Verification items for the finished model (mm, model axes). A direction names the side the tool comes from. Coordinates: 2 decimals unless noted, no trailing zeros. Order: outer loops, then holes, each group sorted by start corner. A loop starts at its lowest first (then second) coordinate and runs counter-clockwise, first axis right, second up.
Q1. Thickness scan on line 1 (X direction, y = 51, z = 1.8); line 2 (Y direction, x = 12, z = 0.2); line 3 (Y direction, x = 24, z = 1.05). Record the ranges inside material, lowest first.
Q2. Draft check along X on faces 1 (the cylindrical face through (78.084, 57.374, 0.986)), 2 (the cylindrical face through (-73.42, -0.79, 0.99)), 3 (the flat face through (1, 9, 2)). Enter one of: pulls with the +X half, pulls with the -X half, needs draft (parallel to the pull), parting line crosses it, or undercut.
Q3. Cross-section at B-B, the plane y = 51. Record the boundary of the cut face in (x, z), and give its area (3 significant figures).
Q4. Depth check by flat-ended pin: P1, Ø3.5, axis at x = 12.15, y = 85.47, coming from the +Z side; P2, Ø1, axis at y = -68, z = 1.5, coming from the +X side; P3, Ø1, axis at y = 42.5, z = 1, coming from the +X side; P4, Ø3.5, axis at x = -58.16, y = -76.19, coming from the -Z side. Enter the tip coordinate at first touch or a pass-through.
Q5. Cross-section at C-C, the plane z = 0.5. Count the separate pieces of the cut face and the enclosed holes in it, and give its area (3 significant figures).
Q6. Cross-section at A-A, the plane x = 0. Record the boundary of the cut face in (y, z).
Q7. Cross-section at D-D, the plane y = 16. Record the boundary of the cut face in (x, z), and give its area (3 significant figures).
Q8. Set-up check for faces 4 (the cylindrical face through (17.088, -82.073, 1.014)), 5 (the flat face through (-72.61, -74.47, 0.99)): record each of +Z, -Z, +X, -X, +Y, -Y from which the full face is reachable in a straight line by a thin tool's end or side.
from build123d import *

# Parameters (mm, degrees)
SKETCH1_R           = 1.5
SKETCH1_R_2         = 1.25
SKETCH1_R_3         = 2.05
SKETCH1_W           = 4
SKETCH1_H           = 23
BOSS_EXTRUDE1_DEPTH = 2
FILLET7_R           = 8
BOSS_EXTRUDE2_DEPTH = 2
FILLET8_R           = 10
SKETCH5_R           = 1.55
CUT_EXTRUDE1_DEPTH  = 10
CUT_EXTRUDE2_DEPTH  = 10
SKETCH8_R           = 1.3
CUT_EXTRUDE4_DEPTH  = 10


with BuildPart() as part:
    # Sketch1 → Boss-Extrude1 (new body)
    with BuildSketch(Plane.XY):
        with BuildLine():
            Line((-86.974134086, 60.104076401), (-60.104076401, 86.974134086))
            Line((-60.104076401, 86.974134086), (60.104076401, 86.974134086))
            Line((60.104076401, 86.974134086), (86.974134086, 60.104076401))
            ThreePointArc((86.974134086, 60.104076401), (73.41582025, 0), (86.974134086, -60.104076401))
            Line((86.974134086, -60.104076401), (60.104076401, -86.974134086))
            Line((60.104076401, -86.974134086), (-60.104076401, -86.974134086))
            Line((-60.104076401, -86.974134086), (-86.974134086, -60.104076401))
            ThreePointArc((-86.974134086, -60.104076401), (-73.41582025, 0), (-86.974134086, 60.104076401))
        make_face()
        with Locations((-15, 57.5)):
            Circle(SKETCH1_R, mode=Mode.SUBTRACT)
        with Locations((-15, 27.5)):
            Circle(SKETCH1_R, mode=Mode.SUBTRACT)
        with Locations((15, 27.5)):
            Circle(SKETCH1_R, mode=Mode.SUBTRACT)
        with Locations((15, 57.5)):
            Circle(SKETCH1_R, mode=Mode.SUBTRACT)
        with Locations((-24, -13.5)):
            Circle(SKETCH1_R_2, mode=Mode.SUBTRACT)
        with Locations((24, -13.5)):
            Circle(SKETCH1_R_2, mode=Mode.SUBTRACT)
        with Locations((24, -46.5)):
            Circle(SKETCH1_R_2, mode=Mode.SUBTRACT)
        with Locations((-24, -46.5)):
            Circle(SKETCH1_R_2, mode=Mode.SUBTRACT)
        with Locations((-76.190755673, 58.159532753)):
            Circle(SKETCH1_R_3, mode=Mode.SUBTRACT)
        with Locations((-58.159532753, 76.190755673)):
            Circle(SKETCH1_R_3, mode=Mode.SUBTRACT)
        with Locations((76.190755673, -58.159532753)):
            Circle(SKETCH1_R_3, mode=Mode.SUBTRACT)
        with Locations((58.159532753, -76.190755673)):
            Circle(SKETCH1_R_3, mode=Mode.SUBTRACT)
        with Locations((-58.159532753, -76.190755673)):
            Circle(SKETCH1_R_3, mode=Mode.SUBTRACT)
        with Locations((-76.190755673, -58.159532753)):
            Circle(SKETCH1_R_3, mode=Mode.SUBTRACT)
        with Locations((58.159532753, 76.190755673)):
            Circle(SKETCH1_R_3, mode=Mode.SUBTRACT)
        with Locations((76.190755673, 58.159532753)):
            Circle(SKETCH1_R_3, mode=Mode.SUBTRACT)
        with Locations((-37, 42.5)):
            Rectangle(SKETCH1_W, SKETCH1_H, mode=Mode.SUBTRACT)
        with Locations((37, 42.5)):
            Rectangle(SKETCH1_W, SKETCH1_H, mode=Mode.SUBTRACT)
        with Locations((37, -30)):
            Rectangle(SKETCH1_W, SKETCH1_H, mode=Mode.SUBTRACT)
        with Locations((-37, -30)):
            Rectangle(SKETCH1_W, SKETCH1_H, mode=Mode.SUBTRACT)
    extrude(amount=BOSS_EXTRUDE1_DEPTH)

    # Fillet7
    fillet7_edges = [part.edges().sort_by_distance(p)[0] for p in [
        (86.974134086, -60.104076401, 1),
        (60.104076401, -86.974134086, 1),
        (-60.104076401, -86.974134086, 1),
        (-86.974134086, -60.104076401, 1),
        (-86.974134086, 60.104076401, 1),
        (-60.104076401, 86.974134086, 1),
        (60.104076401, 86.974134086, 1),
        (86.974134086, 60.104076401, 1),
    ]]
    fillet(fillet7_edges, radius=FILLET7_R)

    # Sketch2 → Boss-Extrude2 (add)
    with BuildSketch(Plane.XY.offset(2)):
        with BuildLine():
            Line((-62.447222151, 84.630988335), (-45.104076401, 101.974134086))
            Line((-45.104076401, 101.974134086), (45.104076401, 101.974134086))
            Line((45.104076401, 101.974134086), (62.447222151, 84.630988335))
            ThreePointArc((62.447222151, 84.630988335), (59.851835361, 86.365170346), (56.790367902, 86.974134086))
            Line((56.790367902, 86.974134086), (-56.790367902, 86.974134086))
            ThreePointArc((-56.790367902, 86.974134086), (-59.851835361, 86.365170346), (-62.447222151, 84.630988335))
        make_face()
    extrude(amount=-BOSS_EXTRUDE2_DEPTH)

    # Fillet8
    fillet8_edges = [part.edges().sort_by_distance(p)[0] for p in [
        (-45.104076401, 101.974134086, 1),
        (45.104076401, 101.974134086, 1),
    ]]
    fillet(fillet8_edges, radius=FILLET8_R)

    # Sketch5 → Cut-Extrude1 (cut)
    with BuildSketch(Plane.XY.offset(2)):
        with Locations((49, 22.5)):
            Circle(SKETCH5_R)
        with Locations((49, -22.5)):
            Circle(SKETCH5_R)
        with Locations((-49, -22.5)):
            Circle(SKETCH5_R)
        with Locations((-49, 22.5)):
            Circle(SKETCH5_R)
    extrude(amount=-CUT_EXTRUDE1_DEPTH, mode=Mode.SUBTRACT)

    # Sketch6 → Cut-Extrude2 (cut)
    with BuildSketch(Plane.XY.offset(2)):
        with BuildLine():
            Line((-30, -62.074134086), (-30, -78.074134086))
            ThreePointArc((-30, -78.074134086), (-34, -82.074134086), (-38, -78.074134086))
            Line((-38, -78.074134086), (-38, -62.074134086))
            ThreePointArc((-38, -62.074134086), (-34, -58.074134086), (-30, -62.074134086))
        make_face()
        with BuildLine():
            Line((-13, -62.074134086), (-13, -78.074134086))
            ThreePointArc((-13, -78.074134086), (-17, -82.074134086), (-21, -78.074134086))
            Line((-21, -78.074134086), (-21, -62.074134086))
            ThreePointArc((-21, -62.074134086), (-17, -58.074134086), (-13, -62.074134086))
        make_face()
        with BuildLine():
            Line((4, -62.074134086), (4, -78.074134086))
            ThreePointArc((4, -78.074134086), (0, -82.074134086), (-4, -78.074134086))
            Line((-4, -78.074134086), (-4, -62.074134086))
            ThreePointArc((-4, -62.074134086), (0, -58.074134086), (4, -62.074134086))
        make_face()
        with BuildLine():
            Line((21, -62.074134086), (21, -78.074134086))
            ThreePointArc((21, -78.074134086), (17, -82.074134086), (13, -78.074134086))
            Line((13, -78.074134086), (13, -62.074134086))
            ThreePointArc((13, -62.074134086), (17, -58.074134086), (21, -62.074134086))
        make_face()
        with BuildLine():
            Line((38, -62.074134086), (38, -78.074134086))
            ThreePointArc((38, -78.074134086), (34, -82.074134086), (30, -78.074134086))
            Line((30, -78.074134086), (30, -62.074134086))
            ThreePointArc((30, -62.074134086), (34, -58.074134086), (38, -62.074134086))
        make_face()
    extrude(amount=-CUT_EXTRUDE2_DEPTH, mode=Mode.SUBTRACT)

    # Sketch8 → Cut-Extrude4 (cut)
    with BuildSketch(Plane.XY.offset(2)):
        with Locations((12.15, 97.474134086)):
            Circle(SKETCH8_R)
        with Locations((12.15, 85.474134086)):
            Circle(SKETCH8_R)
        with Locations((-12.15, 85.474134086)):
            Circle(SKETCH8_R)
        with Locations((-12.15, 97.474134086)):
            Circle(SKETCH8_R)
    extrude(amount=-CUT_EXTRUDE4_DEPTH, mode=Mode.SUBTRACT)


solid = part.part
Check values:
1. line 1: x = -83.04 to -39, -35 to 35, 39 to 83.04
1. line 2: y = -86.97 to 84.18, 86.77 to 96.18, 98.77 to 101.97
1. line 3: y = -86.97 to -47.75, -45.25 to -14.75, -12.25 to 101.97
2. face 1: undercut
2. face 2: pulls with the -X half
2. face 3: needs draft
3. outline: (-83.04, 0) - (-39, 0) - (-39, 2) - (-83.04, 2) - close; (-35, 0) - (35, 0) - (35, 2) - (-35, 2) - close; (39, 0) - (83.04, 0) - (83.04, 2) - (39, 2) - close
3. area: 316 mm2
4. P1: stops at z = 2
4. P2: stops at x = 79.58
4. P3: stops at x = 80.18
4. P4: passes through
5. separate pieces: 1
5. enclosed holes: 33
5. area: 26,700 mm2
6. outline: (-86.97, 0) - (-82.07, 0) - (-82.07, 2) - (-86.97, 2) - close; (-58.07, 0) - (101.97, 0) - (101.97, 2) - (-58.07, 2) - close
7. outline: (-74.33, 0) - (74.33, 0) - (74.33, 2) - (-74.33, 2) - close
7. area: 297 mm2
8. face 4: +Z, -Z
8. face 5: +Z, -Z, -X, -Y
